For this review, take the finished solid that the model builds, in its own axes (mm). A direction names the side the tool comes from. Coordinates: 2 decimals unless noted, no trailing zeros. Order: outer loops, then holes, each group sorted by start corner. A loop starts at its lowest first (then second) coordinate and runs counter-clockwise, first axis right, second up. Notation, with made-up numbers: (44, -35.5) - (52, -35.5) arc R31 ccw to (52, -1.5) - close; hole circle Ø10 at (69, 87). An arc over 180 degrees is marked (long way). One line per item, written item: value. Start each with the question number.
(1) Consider section D-D on z = -16. Write out the cut boundary in (x, y).
(2) Consider section A-A on z = 0. Write out the cut boundary in (x, y).
(3) For faces 1 (the cylindrical face through (7.4, -2.17, 9.76)), 2 (the flat face through (-75, 0, 0)), 3 (the flat face through (-60, 9, -5)), list the 3-axis set-ups (+Z, -Z, +X, -X, +Y, -Y) from which the entire face can be reached by the end or side of a thin tool; tool diameter is ignored.
(4) Clearance check with flat-ended pins moving along their axes: pin 1 (1.5 mm diameter, centred on y = -13.5, z = -16, fed in from -X); pin 2 (4 mm diameter, centred on y = -16, z = -1.5, fed in from +X); pin 3 (1.5 mm diameter, centred on x = -25, z = 3.5, fed in from +Y); pin 4 (12 mm diameter, centred on x = -46.5, z = 4.5, fed in from +Y). State where each tip first meets the part, or that it passes through.
(5) To check wall thickness, follow line 1 along X through (y, z) = (-11, -13.5); line 2 along Y through (x, z) = (-12.5, 0); line 3 along Y through (x, z) = (-35, 17.5). State the ranges of each line that lie inside material, in increasing order.
(6) Consider section C-C on x = -52. Write out the cut boundary in (y, z).
Autodesk Inventor part; units mm, degrees
ref_plane "YZ Plane" through (0, 0, 0) normal (1, 0, 0) x (0, 1, 0)
ref_plane "XZ Plane" through (0, 0, 0) normal (0, 1, 0) x (-1, 0, 0)
ref_plane "XY Plane" through (0, 0, 0) normal (0, 0, 1) x (1, 0, 0)
sketch "Sketch2" plane through (0, 0, 0) normal (1, 0, 0) x (0, 1, 0)
  circle A0 centre (0, 0) radius 10
  dimension "d5" = 20
extrude "Extrusion2" add sketch "Sketch2" along normal blind 15
sketch "Sketch3" plane through (0, 0, 0) normal (-1, 0, 0) x (0, 0, 1)
  circle A0 centre (0, 0) radius 20
  dimension "d8" = 40
extrude "Extrusion3" add sketch "Sketch3" along normal blind 90
sketch "Sketch4" plane through (-90, 0, 0) normal (-1, 0, 0) x (0, 0, 1)
  circle A0 centre (0, 0) radius 20
  circle A1 centre (0, 0) radius 10
  circle A2 centre (0, 0) radius 10
  circle A3 centre (0, 0) radius 20
  dimension "d11" = 20
  dimension "d12" = 40
extrude "Extrusion4" cut sketch "Sketch4" against normal blind 30
sketch "Sketch5" plane through (-90, 0, 0) normal (-1, 0, 0) x (0, 0, 1)
  circle A0 centre (0, 0) radius 10
extrude "Extrusion5" cut sketch "Sketch5" against normal blind 15
equation "\"BendRadius\" = Thickness"
equation "\"BendReliefWidth\" = Thickness"
equation "\"BendReliefDepth\" = 0.5 * Thickness"
equation "\"CornerReliefSize\" = 4 * Thickness"
equation "\"MinimumRemnant\" = 2 * Thickness"
equation "\"TransitionRadius\" = BendRadius"
equation "\"JacobiRadiusSize\" = BendRadius"
equation "\"GapSize\" = Thickness"
properties part number "pin2vathmida" material "Bronze, Soft Tin"
Geometry check:
1. outline: (-60, -12) - (0, -12) - (0, 12) - (-60, 12) - close
2. outline: (-75, -10) - (-60, -10) - (-60, -20) - (0, -20) - (0, -10) - (15, -10) - (15, 10) - (0, 10) - (0, 20) - (-60, 20) - (-60, 10) - (-75, 10) - close
3. face 1: +X
3. face 2: +Z, -Z, -X, +Y, -Y
3. face 3: -X
4. pin 1: passes through
4. pin 2: stops at x = 0
4. pin 3: stops at y = 19.81
4. pin 4: stops at y = 20
5. line 1: x = -60 to 0
5. line 2: y = -20 to 20
5. line 3: y = -9.68 to 9.68
6. outline: circle Ø40 at (0, 0)
